Could you check a few things on this model? Use its own coordinates, in mm. A direction names the side the tool comes from. Coordinates: 2 decimals unless noted, no trailing zeros. Write each loop counter-clockwise with the first axis right and the second up, starting at its lowest first coordinate (ties: lowest second). Pieces come first, ordered by that corner, then holes.
```python
from build123d import *

# Parameters (mm, degrees)
CUT_EXTRUDE1_DEPTH      = 10
CUT_EXTRUDE1_DEPTH_BACK = 10
SKETCH3_W               = 1.5
SKETCH3_H               = 1


with BuildPart() as part:
    # Sketch1 → Revolve1 (revolve)
    with BuildSketch(Plane.YZ, mode=Mode.PRIVATE) as revolve1_sk:
        with BuildLine():
            Line((0, 7), (3, 7))
            ThreePointArc((3, 7), (3.707106781, 6.707106781), (4, 6))
            Line((4, 6), (4, 5))
            Line((4, 5), (2.5, 5))
            Line((2.5, 5), (2.5, -5))
            Line((2.5, -5), (4, -5))
            Line((4, -5), (4, -6))
            ThreePointArc((4, -6), (3.707106781, -6.707106781), (3, -7))
            Line((3, -7), (0, -7))
            Line((0, -7), (0, 7))
        make_face()
    revolve(revolve1_sk.sketch.rotate(Axis((0, 0, 9.31839629), (0, 0, -1)), 180), axis=Axis((0, 0, 9.31839629), (0, 0, -1)))

    # Sketch3 → Cut-Extrude1 (cut, two sides: drawn at the far end of the back side and taken through both)
    with BuildSketch(Plane.YZ.offset(-CUT_EXTRUDE1_DEPTH_BACK)):
        with Locations((0, 6.5)):
            Rectangle(SKETCH3_W, SKETCH3_H)
        with Locations((0, -6.5)):
            Rectangle(SKETCH3_W, SKETCH3_H)
    extrude(amount=CUT_EXTRUDE1_DEPTH + CUT_EXTRUDE1_DEPTH_BACK, mode=Mode.SUBTRACT)


solid = part.part
```
1. I want a section at A-A on x = 0. Please give me the cut outline in (y, z).
Verdict:
outline: (-4, -6) arc R1 ccw to (-3, -7) - (-0.75, -7) - (-0.75, -6) - (0.75, -6) - (0.75, -7) - (3, -7) arc R1 ccw to (4, -6) - (4, -5) - (2.5, -5) - (2.5, 5) - (4, 5) - (4, 6) arc R1 ccw to (3, 7) - (0.75, 7) - (0.75, 6) - (-0.75, 6) - (-0.75, 7) - (-3, 7) arc R1 ccw to (-4, 6) - (-4, 5) - (-2.5, 5) - (-2.5, -5) - (-4, -5) - close
2. Please list where these lines run through material, in increasing order: line 1 along Z through (x, y) = (-1.5, -2.5); line 2 along Z through (x, y) = (-0.75, -0.25); line 3 along Z through (x, y) = (2, -3.25).
Verdict:
line 1: z = -7 to -5, 5 to 7
line 2: z = -6 to 6
line 3: z = -6.58 to -5, 5 to 6.58
3. I want a section at B-B on y = 0. Please give me the cut outline in (x, z).
Verdict:
outline: (-4, -6) - (4, -6) - (4, -5) - (2.5, -5) - (2.5, 5) - (4, 5) - (4, 6) - (-4, 6) - (-4, 5) - (-2.5, 5) - (-2.5, -5) - (-4, -5) - close
4. On a 3-axis mill with a long thin cutter (end or side, diameter ignored), from which of +Z, -Z, +X, -X, +Y, -Y can I reach the whole of each face in a straight line? I mean faces 1 (the face through (3.905, 0.867, -5.507)), 2 (the face through (-2, -2, 5)), 3 (the face through (0, 0, 6)), 4 (the face through (0, 0, -6)). Say none if no direction works.
Verdict:
face 1: +Z, -Z
face 2: none
face 3: +Z, +X, -X
face 4: -Z, +X, -X
5. For pin 1 (0.8 mm diameter, centred on x = -1.5, y = 0, fed in from +Z); pin 2 (3 mm diameter, centred on x = 0, z = -3, fed in from +Y); pin 3 (1 mm diameter, centred on y = 1, z = -2, fed in from +X), each with a flat end and sliding along its axis, tell me the tip position at first contact or that it passes through.
Verdict:
pin 1: stops at z = 6
pin 2: stops at y = 2.5
pin 3: stops at x = 2.45
6. I want a section at C-C on z = 3. Please give me the cut outline in (x, y).
Verdict:
outline: circle Ø5 at (0, 0)
7. I want a section at D-D on z = -5.25. Please give me the cut outline in (x, y).
Verdict:
outline: circle Ø8 at (0, 0)
8. If we mould it in two halves opening along Y, with no side actions, what happens to faces 5 (the face through (-0.1, 2.5, -0.1)), 6 (the face through (-0.1, -0.75, 6.5)), 7 (the face through (-2, 2, -5))? For each: pulls with the +Y half, pulls with the -Y half, needs draft (parallel to the pull), parting line crosses it, or undercut.
Verdict:
face 5: parting line crosses it
face 6: undercut
face 7: needs draft
